Source: CAD feature listing. Evaluate the final solid. Frame: model axes, mm. Face numbers are marked on the shaded views. Give positions to 0.01 mm unless a question says otherwise; leave off trailing zeros. Loops run counter-clockwise (first coordinate to the right, second up) from the corner with the lowest first, then second, coordinate; pieces in that order, holes last. Notation, with made-up numbers: (71, 67.25) -> (124, 67.25) arc R26 cw to (124, 89.25) -> close; hole circle Ø10 at (3, -7.5). An arc over 180 degrees is marked (long way). Answer as a JSON object with one key per item and string values. Group by question number.
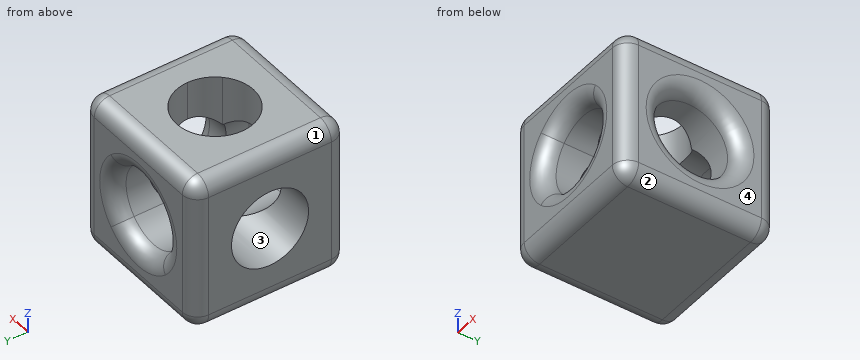
from build123d import *

# Parameters (mm, degrees)
F1_DEPTH = 50.8
F3_R     = 12.7614495694
F4_DEPTH = 50.8
F5_DEPTH = 25.4
F6_R     = 5.08


with BuildPart() as f1:
    # F0 (on Front) → F1 (new body)
    with BuildSketch(Plane.XZ):
        with BuildLine():
            Line((0, 50.8000037167), (0, 0))
            Line((0, 0), (16.4197442074, 16.4197454088))
            ThreePointArc((16.4197442074, 16.4197454088), (12.7, 25.4000018583), (16.4197442074, 34.3802583079))
            Line((16.4197442074, 34.3802583079), (0, 50.8000037167))
        make_face()
        with BuildLine():
            Line((50.8, 50.8000037167), (0, 50.8000037167))
            Line((0, 50.8000037167), (16.4197442074, 34.3802583079))
            ThreePointArc((16.4197442074, 34.3802583079), (25.4, 38.1000018583), (34.3802557926, 34.3802583079))
            Line((34.3802557926, 34.3802583079), (50.8, 50.8000037167))
        make_face()
        with BuildLine():
            Line((34.3802557926, 16.4197454088), (50.8, 0))
            Line((50.8, 0), (50.8, 50.8000037167))
            Line((50.8, 50.8000037167), (34.3802557926, 34.3802583079))
            ThreePointArc((34.3802557926, 34.3802583079), (37.133269974, 30.260081664), (38.1, 25.4000018583))
            ThreePointArc((38.1, 25.4000018583), (37.133269974, 20.5399220527), (34.3802557926, 16.4197454088))
        make_face()
        with BuildLine():
            Line((16.4197442074, 16.4197454088), (0, 0))
            Line((0, 0), (50.8, 0))
            Line((50.8, 0), (34.3802557926, 16.4197454088))
            ThreePointArc((34.3802557926, 16.4197454088), (25.4, 12.7000018583), (16.4197442074, 16.4197454088))
        make_face()
    extrude(amount=F1_DEPTH)

    # F3 (on face) → F4 (cut)
    with BuildSketch(Plane.YZ.offset(50.8)):
        with Locations((-25.4, 25.4000018583)):
            Circle(F3_R)
    extrude(amount=-F4_DEPTH, mode=Mode.SUBTRACT)

    # F2 (on face) → F5 (cut)
    with BuildSketch(Plane.XY.offset(50.8000037167)):
        with BuildLine():
            ThreePointArc((38.1, -25.4), (37.1332700629, -20.539920409), (34.3802561211, -16.4197438789))
            Line((34.3802561211, -16.4197438789), (25.4, -25.4))
            Line((25.4, -25.4), (34.3802561211, -34.3802561211))
            ThreePointArc((34.3802561211, -34.3802561211), (37.1332700629, -30.260079591), (38.1, -25.4))
        make_face()
        with BuildLine():
            Line((25.4, -25.4), (34.3802561211, -16.4197438789))
            ThreePointArc((34.3802561211, -16.4197438789), (25.4, -12.7), (16.4197438789, -16.4197438789))
            Line((16.4197438789, -16.4197438789), (25.4, -25.4))
        make_face()
        with BuildLine():
            Line((34.3802561211, -34.3802561211), (25.4, -25.4))
            Line((25.4, -25.4), (16.4197438789, -34.3802561211))
            ThreePointArc((16.4197438789, -34.3802561211), (25.4, -38.1), (34.3802561211, -34.3802561211))
        make_face()
        with BuildLine():
            Line((16.4197438789, -34.3802561211), (25.4, -25.4))
            Line((25.4, -25.4), (16.4197438789, -16.4197438789))
            ThreePointArc((16.4197438789, -16.4197438789), (12.7, -25.4), (16.4197438789, -34.3802561211))
        make_face()
    extrude(amount=-F5_DEPTH, mode=Mode.SUBTRACT)

    # F6
    f6_edges = [f1.edges().sort_by_distance(p)[0] for p in [
        (0, -25.4, 50.800004),
        (0, -50.8, 25.400002),
        (50.8, -50.8, 25.400002),
        (50.8, 0, 25.400002),
        (50.8, -25.4, 50.800004),
        (50.8, -25.4, 0),
        (50.8, -38.16145, 25.400002),
        (25.4, -50.8, 0),
        (25.4, -50.8, 50.800004),
        (16.419744, -50.8, 34.380258),
        (0, -25.4, 0),
        (0, 0, 25.400002),
        (25.4, 0, 50.800004),
        (25.4, 0, 0),
        (16.419744, 0, 34.380258),
    ]]
    fillet(f6_edges, radius=F6_R)


solid = f1.part
(1) Material intervals for line 1 (Z direction, x = 39.5, y = -26); line 2 (Z direction, x = 22, y = -25.4); line 3 (X direction, y = -5, z = 12.5), sorted ascending. Write a range as from..to.
(2) First-contact query: pin 1 (1.5 mm diameter, centred on x = 33.5, z = 35, fed in from +Y); pin 2 (10 mm diameter, centred on x = 14, z = 14.5, fed in from -Y); pin 3 (4 mm diameter, centred on x = 36, z = 21, fed in from +Y); pin 4 (5 mm diameter, centred on x = 17, z = 27, fed in from +Y). Flat tips, straight axial feed; report the tip coordinate or a pass-through.
(3) Section query A-A on x = 6.5. Return the cut outline in (y, z), plus the area to 3 significant figures.
(4) Mould query, pull axis Z, two halves, no side actions, for the marked faces 1, 2, 3 and 4. Classes: pulls with the +Z half, pulls with the -Z half, needs draft (parallel to the pull), parting line crosses it, or undercut.
(5) Section query B-B on z = 18.5. State how many separate pieces and enclosed holes the cut face has, plus the area to 3 significant figures.
Result:
{
 "1": {"line 1": "0..12.65, 38.15..50.8", "line 2": "0..12.64", "line 3": "0..50.8"},
 "2": {"pin 1": "y = -2.67", "pin 2": "y = -50.8", "pin 3": "y = -2.38", "pin 4": "through"},
 "3": {"outline": "(-50.8, 5.08) arc R5.08 ccw to (-45.72, 0) -> (-5.08, 0) arc R5.08 ccw to (0, 5.08) -> (0, 45.72) arc R5.08 ccw to (-5.08, 50.8) -> (-45.72, 50.8) arc R5.08 ccw to (-50.8, 45.72) -> close; hole circle Ø25.52 at (-25.4, 25.4)", "area": "2,050 mm²"},
 "4": {"face 1": "pulls with the +Z half", "face 2": "pulls with the -Z half", "face 3": "undercut", "face 4": "needs draft"},
 "5": {"separate pieces": "4", "enclosed holes": "0", "area": "804 mm²"}
}
